from build123d import *

# Parameters (mm, degrees)
F1_DEPTH    = 15
F4_T1_DEPTH = 20.1961524227
F5_START    = 6.5
F5_DEPTH    = 2
F6_START    = 4.5
F6_DEPTH    = 2
F7_START    = 8.5
F7_DEPTH    = 2
F8_START    = 2.5
F8_DEPTH    = 2
F9_START    = 6.5
F9_DEPTH    = 2
F10_START   = 10.5
F10_DEPTH   = 2


# Not quite as in the source:
# - a fillet or chamfer that OpenCascade refuses, or shapes differently, is made with other operations: its cross-section is extruded or revolved along the edge and cut away or added
# - an extrude whose draft closes it to a point is written as a loft to that point
# - a feature names something its author has since deleted; it is built from what else it names


with BuildPart() as f1:
    # F0 (on Right) → F1 (new body)
    with BuildSketch(Plane.YZ):
        with BuildLine():
            Line((4.25, 2.1650635095), (6.25, 2.1650635095))
            Line((6.25, 2.1650635095), (5.25, 3.897114317))
            ThreePointArc((5.25, 3.897114317), (4.5179491924, 3.1650635095), (4.25, 2.1650635095))
        make_face()
        with BuildLine():
            ThreePointArc((4.25, 2.1650635095), (4.5179491924, 3.1650635095), (5.25, 3.897114317))
            Line((5.25, 3.897114317), (1, 11.2583302492))
            ThreePointArc((1, 11.2583302492), (0, 10.9903810568), (-1, 11.2583302492))
            Line((-1, 11.2583302492), (-5.25, 3.897114317))
            ThreePointArc((-5.25, 3.897114317), (-4.5179491924, 3.1650635095), (-4.25, 2.1650635095))
            Line((-4.25, 2.1650635095), (4.25, 2.1650635095))
        make_face()
        with BuildLine():
            ThreePointArc((-1, 11.2583302492), (0, 10.9903810568), (1, 11.2583302492))
            Line((1, 11.2583302492), (0, 12.9903810568))
            Line((0, 12.9903810568), (-1, 11.2583302492))
        make_face()
        with BuildLine():
            Line((-6.25, 2.1650635095), (-4.25, 2.1650635095))
            ThreePointArc((-4.25, 2.1650635095), (-4.5179491924, 3.1650635095), (-5.25, 3.897114317))
            Line((-5.25, 3.897114317), (-6.25, 2.1650635095))
        make_face()
    extrude(amount=F1_DEPTH)

    # F1_face (on face) → F2 section 0
    with BuildSketch(Plane(origin=(0, 0, 5.7735026919), x_dir=(0, 1, 0), z_dir=(-1, 0, 0)), mode=Mode.PRIVATE) as f2_s0:
        Polygon((0, -7.2168783649), (6.25, 3.6084391824), (-6.25, 3.6084391824), align=None)
    loft([f2_s0.sketch, Vertex(-3.6084391824, 0, 5.7735026919)], ruled=True)

    # F1_face1 (on face) → F3 section 0
    with BuildSketch(Plane(origin=(15, 0, 5.7735026919), x_dir=(0, 1, 0), z_dir=(1, 0, 0)), mode=Mode.PRIVATE) as f3_s0:
        Polygon((6.25, -3.6084391824), (0, 7.2168783649), (-6.25, -3.6084391824), align=None)
    loft([f3_s0.sketch, Vertex(18.6084391824, 0, 5.7735026919)], ruled=True)

    # F4: fillet of radius 0.6 on 3 edges, made by hand

    # F4_s2 → F4_t1 (cut)
    with BuildSketch(Plane.YZ.offset(-2.5980762114)):
        with BuildLine():
            ThreePointArc((0.5196152423, 12.0903810568), (0, 12.3903810568), (-0.5196152423, 12.0903810568))
            Line((-0.5196152423, 12.0903810568), (0, 12.9903810568))
            Line((0, 12.9903810568), (0.5196152423, 12.0903810568))
        make_face()
        with BuildLine():
            ThreePointArc((-5.2107695155, 2.1650635095), (-5.7303847577, 2.4650635095), (-5.7303847577, 3.0650635095))
            Line((-5.7303847577, 3.0650635095), (-6.25, 2.1650635095))
            Line((-6.25, 2.1650635095), (-5.2107695155, 2.1650635095))
        make_face()
        with BuildLine():
            ThreePointArc((5.7303847577, 3.0650635095), (5.7303847577, 2.4650635095), (5.2107695155, 2.1650635095))
            Line((5.2107695155, 2.1650635095), (6.25, 2.1650635095))
            Line((6.25, 2.1650635095), (5.7303847577, 3.0650635095))
        make_face()
    extrude(amount=F4_T1_DEPTH, mode=Mode.SUBTRACT)

    # F0 (on Right) → F5 (cut)
    with BuildSketch(Plane.YZ.offset(F5_START)):
        with BuildLine():
            ThreePointArc((-1, 11.2583302492), (0, 10.9903810568), (1, 11.2583302492))
            Line((1, 11.2583302492), (0, 12.9903810568))
            Line((0, 12.9903810568), (-1, 11.2583302492))
        make_face()
    extrude(amount=F5_DEPTH, mode=Mode.SUBTRACT)

    # F0 (on Right) → F6 (cut)
    with BuildSketch(Plane.YZ.offset(F6_START)):
        with BuildLine():
            Line((-6.25, 2.1650635095), (-4.25, 2.1650635095))
            ThreePointArc((-4.25, 2.1650635095), (-4.5179491924, 3.1650635095), (-5.25, 3.897114317))
            Line((-5.25, 3.897114317), (-6.25, 2.1650635095))
        make_face()
    extrude(amount=F6_DEPTH, mode=Mode.SUBTRACT)

    # F0 (on Right) → F7 (cut)
    with BuildSketch(Plane.YZ.offset(F7_START)):
        with BuildLine():
            Line((-6.25, 2.1650635095), (-4.25, 2.1650635095))
            ThreePointArc((-4.25, 2.1650635095), (-4.5179491924, 3.1650635095), (-5.25, 3.897114317))
            Line((-5.25, 3.897114317), (-6.25, 2.1650635095))
        make_face()
    extrude(amount=F7_DEPTH, mode=Mode.SUBTRACT)

    # F0 (on Right) → F8 (cut)
    with BuildSketch(Plane.YZ.offset(F8_START)):
        with BuildLine():
            Line((4.25, 2.1650635095), (6.25, 2.1650635095))
            Line((6.25, 2.1650635095), (5.25, 3.897114317))
            ThreePointArc((5.25, 3.897114317), (4.5179491924, 3.1650635095), (4.25, 2.1650635095))
        make_face()
    extrude(amount=F8_DEPTH, mode=Mode.SUBTRACT)

    # F0 (on Right) → F9 (cut)
    with BuildSketch(Plane.YZ.offset(F9_START)):
        with BuildLine():
            Line((4.25, 2.1650635095), (6.25, 2.1650635095))
            Line((6.25, 2.1650635095), (5.25, 3.897114317))
            ThreePointArc((5.25, 3.897114317), (4.5179491924, 3.1650635095), (4.25, 2.1650635095))
        make_face()
    extrude(amount=F9_DEPTH, mode=Mode.SUBTRACT)

    # F0 (on Right) → F10 (cut)
    with BuildSketch(Plane.YZ.offset(F10_START)):
        with BuildLine():
            Line((4.25, 2.1650635095), (6.25, 2.1650635095))
            Line((6.25, 2.1650635095), (5.25, 3.897114317))
            ThreePointArc((5.25, 3.897114317), (4.5179491924, 3.1650635095), (4.25, 2.1650635095))
        make_face()
    extrude(amount=F10_DEPTH, mode=Mode.SUBTRACT)


solid = f1.part
Geometry: final body of the model. Coordinates: model frame, mm. A direction names the side the tool comes from. Give positions to 0.01 mm unless a question says otherwise; leave off trailing zeros. Write each loop counter-clockwise with the first axis right and the second up, starting at its lowest first coordinate (ties: lowest second). Pieces come first, ordered by that corner, then holes. Notation, with made-up numbers: (25.5, 5) - (63.5, 5) arc R22 cw to (63.5, 14) - close; hole circle Ø6 at (68.25, 53.5). An arc over 180 degrees is marked (long way). Return JSON: item names as keys, results as strings. Group by question number.
1) Section B-B on y = -4.5. Return the cut outline in (x, z), plus the area to 3 significant figures.
2) Section D-D on x = 13.75. Return the cut outline in (y, z), plus the area to 3 significant figures.
3) Section C-C on z = 7. Return the cut outline in (x, y).
4) First-contact query: P1, Ø1.1, axis at y = -0.5, z = 11.5, coming from the +X side; P2, Ø0.8, axis at y = 5, z = 3.5, coming from the -X side; P3, Ø1.5, axis at x = 11, y = 1.5, coming from the +Z side. Flat tips, straight axial feed; report the tip coordinate or a pass-through.
5) Mould query, pull axis X, two halves, no side actions, for faces 1 (the cylindrical face through (9.486, 5.735, 2.473)), 2 (the flat face through (8.5, 0, 12)), 3 (the flat face through (16.43, 1.93, 6.79)). Classes: released by +X, released by -X, zero draft, split by the parting line, or undercut.
6) Section A-A on x = 3.75. Return the cut outline in (y, z).
7) Line query: line 1 (X direction, y = 4.75, z = 3); line 2 (Z direction, x = 13.5, y = -1.5); line 3 (Y direction, x = 10.75, z = 3.5). Output: solid intervals per line, ascending.
8) Set-up query: faces 4 (the flat face through (6.5, 0, 12)), 5 (the flat face through (6.5, -5, 3)), 6 (the flat face through (10.5, 5, 3)). Return all of +Z, -Z, +X, -X, +Y, -Y with unobstructed straight access to the full face (end or side cutting, diameter ignored); none if empty.
Filled in:
{
 "1": {"outline": "(-1.01, 3.18) - (0, 2.17) - (4.5, 2.17) - (4.5, 3.13) - (6.5, 3.13) - (6.5, 2.17) - (8.5, 2.17) - (8.5, 3.13) - (10.5, 3.13) - (10.5, 2.17) - (15, 2.17) - (16.01, 3.18) - (15, 5.2) - (0, 5.2) - close", "area": "44.7 mm^2"},
 "2": {"outline": "(-5.73, 3.07) arc R0.6 ccw to (-5.21, 2.17) - (5.21, 2.17) arc R0.6 ccw to (5.73, 3.07) - (0.52, 12.09) arc R0.6 ccw to (-0.52, 12.09) - close", "area": "66.9 mm^2"},
 "3": {"outline": "(-3, 0) - (0, -3.46) - (15, -3.46) - (18, 0) - (15, 3.46) - (0, 3.46) - close"},
 "4": {"P1": "stops at x = 15.86", "P2": "stops at x = -0.82", "P3": "stops at z = 11.69"},
 "5": {"face 1": "zero draft", "face 2": "undercut", "face 3": "released by +X"},
 "6": {"outline": "(-5.73, 3.07) arc R0.6 ccw to (-5.21, 2.17) - (4.25, 2.17) arc R2 cw to (5.25, 3.9) - (0.52, 12.09) arc R0.6 ccw to (-0.52, 12.09) - close"},
 "7": {"line 1": "x = -0.83 to 2.5, 4.5 to 6.5, 8.5 to 10.5, 12.5 to 15.83", "line 2": "z = 2.17 to 10.39", "line 3": "y = -5.48 to 4.76"},
 "8": {"face 4": "+Z", "face 5": "-Z, -Y", "face 6": "-Z, +Y"}
}
